```python
from build123d import *

# Parameters (mm, degrees)
MODEL_W             = 239.114
MODEL_H             = 131.298938207
EXTRUDE_2_DEPTH     = 10
EXTRUDE_3_DEPTH     = 8.5
EXTRUDE_4_DEPTH     = 5
SKETCH_3_R          = 2.5
EXTRUDE_5_DEPTH     = 5
EXTRUDE_5_2_DEPTH   = 5
EXTRUDE_5_3_DEPTH   = 5
EXTRUDE_5_4_DEPTH   = 5
EXTRUDE_6_DEPTH     = 239.114
SKETCH_5_W          = 25
SKETCH_5_H          = 5.998631207
CUT_EXTRUDE_1_DEPTH = 3.5


with BuildPart() as part:
    # Model → Extrude 2 (new body)
    with BuildSketch(Plane.XY):
        with Locations((559.31883528, 226.885059923)):
            Rectangle(MODEL_W, MODEL_H)
        with BuildLine():
            Line((442.76183528, 289.535897819), (675.87583528, 289.535897819))
            Line((675.87583528, 289.535897819), (675.87583528, 217.861297819))
            Line((675.87583528, 217.861297819), (672.87583528, 217.861297819))
            ThreePointArc((672.87583528, 217.861297819), (671.805369011, 217.663814896), (670.87583528, 217.097365797))
            ThreePointArc((670.87583528, 217.097365797), (669.87583528, 214.861297819), (670.87583528, 212.625229842))
            ThreePointArc((670.87583528, 212.625229842), (671.805369011, 212.058780742), (672.87583528, 211.861297819))
            Line((672.87583528, 211.861297819), (675.87583528, 211.861297819))
            Line((675.87583528, 211.861297819), (675.87583528, 164.235590819))
            Line((675.87583528, 164.235590819), (442.76183528, 164.235590819))
            Line((442.76183528, 164.235590819), (442.76183528, 211.861297819))
            Line((442.76183528, 211.861297819), (445.76183528, 211.861297819))
            ThreePointArc((445.76183528, 211.861297819), (446.832301549, 212.058780742), (447.76183528, 212.625229842))
            ThreePointArc((447.76183528, 212.625229842), (448.76183528, 214.861297819), (447.76183528, 217.097365797))
            ThreePointArc((447.76183528, 217.097365797), (446.832301549, 217.663814896), (445.76183528, 217.861297819))
            Line((445.76183528, 217.861297819), (442.76183528, 217.861297819))
            Line((442.76183528, 217.861297819), (442.76183528, 289.535897819))
        make_face(mode=Mode.SUBTRACT)
    extrude(amount=EXTRUDE_2_DEPTH)

    # Model_4 → Extrude 3 (add)
    with BuildSketch(Plane.XY):
        Polygon((445.76183528, 167.235590819), (445.76183528, 211.861297819), (442.76183528, 211.861297819), (442.76183528, 164.235590819), (675.87583528, 164.235590819), (675.87583528, 211.861297819), (672.87583528, 211.861297819), (672.87583528, 167.235590819), align=None)
        Polygon((442.76183528, 217.861297819), (442.76183528, 289.535897819), (675.87583528, 289.535897819), (675.87583528, 217.861297819), (672.87583528, 217.861297819), (672.87583528, 286.535897819), (445.76183528, 286.535897819), (445.76183528, 217.861297819), align=None)
    extrude(amount=EXTRUDE_3_DEPTH)

    # Model_5 → Extrude 4 (add)
    with BuildSketch(Plane.XY):
        with BuildLine():
            ThreePointArc((672.87583528, 211.861297819), (671.805369011, 212.058780742), (670.87583528, 212.625229842))
            Line((670.87583528, 212.625229842), (670.87583528, 169.235590819))
            Line((670.87583528, 169.235590819), (447.76183528, 169.235590819))
            Line((447.76183528, 169.235590819), (447.76183528, 212.625229842))
            ThreePointArc((447.76183528, 212.625229842), (446.832301549, 212.058780742), (445.76183528, 211.861297819))
            Line((445.76183528, 211.861297819), (445.76183528, 167.235590819))
            Line((445.76183528, 167.235590819), (672.87583528, 167.235590819))
            Line((672.87583528, 167.235590819), (672.87583528, 211.861297819))
        make_face()
        with BuildLine():
            ThreePointArc((670.87583528, 217.097365797), (671.805369011, 217.663814896), (672.87583528, 217.861297819))
            Line((672.87583528, 217.861297819), (672.87583528, 286.535897819))
            Line((672.87583528, 286.535897819), (539.76183528, 286.535897819))
            Line((539.76183528, 286.535897819), (514.76183528, 286.535897819))
            Line((514.76183528, 286.535897819), (445.76183528, 286.535897819))
            Line((445.76183528, 286.535897819), (445.76183528, 217.861297819))
            ThreePointArc((445.76183528, 217.861297819), (446.832301549, 217.663814896), (447.76183528, 217.097365797))
            Line((447.76183528, 217.097365797), (447.76183528, 284.535897819))
            Line((447.76183528, 284.535897819), (670.87583528, 284.535897819))
            Line((670.87583528, 284.535897819), (670.87583528, 217.097365797))
        make_face()
    extrude(amount=EXTRUDE_4_DEPTH)



with BuildPart() as body_2:
    # Sketch 3 → Extrude 5 (new body)
    with BuildSketch(Plane(origin=(0, 0, 0), x_dir=(-1, 0, 0), z_dir=(0, 0, -1))):
        with Locations((-577.62472278, 252.961297819)):
            Circle(SKETCH_3_R)
    extrude(amount=-EXTRUDE_5_DEPTH)


with BuildPart() as body_3:
    # Sketch 3 → Extrude 5 2 (new body)
    with BuildSketch(Plane(origin=(0, 0, 0), x_dir=(-1, 0, 0), z_dir=(0, 0, -1))):
        with Locations((-614.53372278, 195.811572819)):
            Circle(SKETCH_3_R)
    extrude(amount=-EXTRUDE_5_2_DEPTH)


with BuildPart() as body_4:
    # Sketch 3 → Extrude 5 3 (new body)
    with BuildSketch(Plane(origin=(0, 0, 0), x_dir=(-1, 0, 0), z_dir=(0, 0, -1))):
        with Locations((-457.84983528, 195.811597819)):
            Circle(SKETCH_3_R)
    extrude(amount=-EXTRUDE_5_3_DEPTH)


with BuildPart() as body_5:
    # Sketch 3 → Extrude 5 4 (new body)
    with BuildSketch(Plane(origin=(0, 0, 0), x_dir=(-1, 0, 0), z_dir=(0, 0, -1))):
        with Locations((-454.62472278, 252.961297819)):
            Circle(SKETCH_3_R)
    extrude(amount=-EXTRUDE_5_4_DEPTH)


with BuildPart() as part_1:
    add(part.part)

    add(body_2.part)  # Extrude 6 merges body 2

    add(body_3.part)  # Extrude 6 merges body 3

    add(body_4.part)  # Extrude 6 merges body 4

    add(body_5.part)  # Extrude 6 merges body 5
    # Sketch 4 → Extrude 6 (add)
    with BuildSketch(Plane.ZY.offset(-439.76183528)):
        Polygon((-9.898975205, 292.535462726), (2.890322341, 48.501128108), (15.872506293, 49.181495539), (10, 161.235590819), (0, 161.235590819), (0, 292.534529026), align=None)
    extrude(amount=-EXTRUDE_6_DEPTH)

    # Sketch 5 → Cut-Extrude 1 (cut)
    with BuildSketch(Plane.XY.offset(8.5)):
        with Locations((527.26183528, 289.535213423)):
            Rectangle(SKETCH_5_W, SKETCH_5_H)
    extrude(amount=-CUT_EXTRUDE_1_DEPTH, mode=Mode.SUBTRACT)


solid = part_1.part
```
The listing builds one solid part. Answer for the finished solid, in the listing's coordinates (mm). A direction names the side the tool comes from. Coordinates: 2 decimals unless noted, no trailing zeros. Loops run counter-clockwise (first coordinate to the right, second up) from the corner with the lowest first, then second, coordinate; pieces in that order, holes last. Notation, with made-up numbers: (66, 29) - (90, 29) arc R28 ccw to (90, 60) - close; hole circle Ø8 at (42.25, 17.5). An arc over 180 degrees is marked (long way). Use a Markdown table: item, result. Add a question column.
1) The part is cut by section B-B, the plane y = 175. Give the vertices of the cut face in (x, z), and give its area (3 significant figures).
2) Given pin 1 (5 mm diameter, centred on x = 577.5, y = 133, fed in from +Z); pin 2 (1 mm diameter, centred on x = 623, y = 101, fed in from -Z); pin 3 (1.2 mm diameter, centred on x = 674, z = 9.5, fed in from -Y), each flat-ended and moving along its own axis, determine where each tip first touches the part or whether it passes through.
3) The mould has two halves that part along X. Classify faces 3 (the flat face through (558, 226, 0)), 4 (the flat face through (678.876, 172, 3)), 5 (the flat face through (559, 164, 10)): released by +X, released by -X, zero draft, split by the parting line, or undercut.
4) The part is cut by section C-C, the plane z = -6. Give the vertices of the cut face in (x, y).
5) The part is cut by section A-A, the plane x = 526. Give the vertices of the cut face in (y, z), and give its area (3 significant figures).
6) The part is cut by section D-D, the plane y = 108. Give the vertices of the cut face in (x, z).
7) For faces 1 (the flat face through (463, 288, 8.5)), 2 (the flat face through (557.645, 48.837, 9.291)), determine the directions among +Z, -Z, +X, -X, +Y, -Y from which every point of the face is accessible in a straight line to the end or side of a thin tool.
8) Find the intervals of material crossed by line 1 (X direction, y = 224.5, z = 5.5); line 2 (X direction, y = 208.5, z = 1.5); line 3 (Y direction, x = 543, z = 9), in increasing order.
Here are the results:
| question | item | result |
|---|---|---|
| 1 | outline | (439.76, -3.74) - (678.88, -3.74) - (678.88, 10) - (675.88, 10) - (675.88, 8.5) - (672.88, 8.5) - (672.88, 5) - (670.88, 5) - (670.88, 0) - (447.76, 0) - (447.76, 5) - (445.76, 5) - (445.76, 8.5) - (442.76, 8.5) - (442.76, 10) - (439.76, 10) - close |
| 1 | area | 1,030 mm^2 |
| 2 | pin 1 | stops at z = 11.61 |
| 2 | pin 2 | stops at z = 0.11 |
| 2 | pin 3 | stops at y = 48.82 |
| 3 | face 3 | undercut |
| 3 | face 4 | released by +X |
| 3 | face 5 | zero draft |
| 4 | outline | (439.76, 218.14) - (678.88, 218.14) - (678.88, 292.54) - (439.76, 292.54) - close |
| 5 | outline | (48.5, 2.89) - (292.54, -9.9) - (292.53, 0) - (292.53, 5) - (284.54, 5) - (284.54, 0) - (169.24, 0) - (169.24, 5) - (167.24, 5) - (167.24, 8.5) - (164.24, 8.5) - (164.24, 10) - (161.24, 10) - (49.18, 15.87) - close; (289.54, 8.5) - (292.53, 8.5) - (292.53, 10) - (289.54, 10) - close |
| 5 | area | 2,420 mm^2 |
| 6 | outline | (439.76, -0.23) - (678.88, -0.23) - (678.88, 12.79) - (439.76, 12.79) - close |
| 7 | face 1 | +Z |
| 7 | face 2 | +Z, +X, -X, -Y |
| 8 | line 1 | x = 439.76 to 445.76, 672.88 to 678.88 |
| 8 | line 2 | x = 439.76 to 447.76, 670.88 to 678.88 |
| 8 | line 3 | y = 48.82 to 164.24, 289.54 to 292.53 |
